The model under review builds one solid part; all positions refer to its coordinate system, in mm. A direction names the side the tool comes from. Round coordinates to 2 decimals unless told otherwise and drop trailing zeros. Loops run counter-clockwise (first coordinate to the right, second up) from the corner with the lowest first, then second, coordinate; pieces in that order, holes last. Notation, with made-up numbers: (-25, -12.75) - (28, -12.75) arc R18 ccw to (28, 20.25) - close; hole circle Ø8 at (3.5, -15). An arc over 180 degrees is marked (long way). Answer as CSV lines item,"result".
from build123d import *

# Parameters (mm, degrees)
FILLET1_R = 1


with BuildPart() as part:
    # Sketch1 → Revolve2 (revolve)
    with BuildSketch(Plane.XY, mode=Mode.PRIVATE) as revolve2_sk:
        with BuildLine():
            Line((12.5, 0), (10, 0))
            ThreePointArc((10, 0), (7.071067812, -7.071067812), (0, -10))
            Line((0, -10), (0, -35))
            Line((0, -35), (5, -35))
            Line((5, -35), (5, -11.456439237))
            ThreePointArc((5, -11.456439237), (10.458250332, -6.846531969), (12.5, 0))
        make_face()
    revolve(revolve2_sk.sketch.rotate(Axis((0, -11.87690577, 0), (0, 1, 0)), 90), axis=Axis((0, -11.87690577, 0), (0, 1, 0)))

    # Fillet1
    fillet1_edges = [part.edges().sort_by_distance(p)[0] for p in [
        (0, -11.456439237, 5),
        (0, -35, 5),
    ]]
    fillet(fillet1_edges, radius=FILLET1_R)


solid = part.part
1. Take a section at B-B (z = 7.25). State the section outline as (x, y) points.
Numbers:
outline,"(-10.18, 0) arc R10.18 ccw to (10.18, 0) - (6.89, 0) arc R6.89 cw to (-6.89, 0) - close"
2. Take a section at A-A (y = -26). State the section outline as (x, z) points.
Numbers:
outline,"circle Ø10 at (0, 0)"
3. Take a section at C-C (y = -3.5). State the section outline as (x, z) points (1 decimal).
Numbers:
outline,"circle Ø24 at (0, 0); hole circle Ø18.7 at (0, 0)"
4. Tool access review of faces 1 (the face through (-10.2, 0, 0.1)), 2 (the face through (-1.5, -22.89, -4.77)): name each direction out of +Z, -Z, +X, -X, +Y, -Y from which nothing blocks a thin tool from reaching the whole face with its end or side.
Numbers:
face 1,"+Z, -Z, +X, -X, +Y"
face 2,"-Y"
5. Clearance check with flat-ended pins moving along their axes: pin 1 (4 mm diameter, centred on y = -18, z = 7.5, fed in from -X); pin 2 (1 mm diameter, centred on x = -3.5, y = -25.5, fed in from -Z); pin 3 (3 mm diameter, centred on x = -3.5, z = -3.5, fed in from +Y); pin 4 (4 mm diameter, centred on x = -6, y = -14.5, fed in from +Z). State where each tip first meets the part, or that it passes through.
Numbers:
pin 1,"passes through"
pin 2,"stops at z = -4"
pin 3,"stops at y = -7.64"
pin 4,"stops at z = 3"
6. Take a section at D-D (x = -7.5). State the section outline as (y, z) points.
Numbers:
outline,"(0, -10) - (0, -6.61) arc R6.61 cw to (0, 6.61) - (0, 10) arc R10 ccw to start"
7. Wall thickness on probe 1 along Z at (x, y) = (-1.5, -1.5); probe 2 along X at (y, z) = (-30.5, 0); probe 3 along Y at (x, z) = (9.25, 0.25): over which ranges is each line inside the solid? List them lowest first.
Numbers:
probe 1,"z = -12.32 to -9.77, 9.77 to 12.32"
probe 2,"x = -5 to 5"
probe 3,"y = -8.4 to -3.79"
